from build123d import *

# Parameters (mm, degrees)
ESBO_O1_W                         = 120
ESBO_O1_H                         = 100
ESBO_O1_R                         = 5
RESSALTO_EXTRUS_O1_DEPTH          = 14
REBAIXO_PARA_SHCS_M81_D           = 9
REBAIXO_PARA_SHCS_M81_CBORE_D     = 14
REBAIXO_PARA_SHCS_M81_CBORE_DEPTH = 9


with BuildPart() as part:
    # Esboço1 → Ressalto-extrusão1 (new body)
    with BuildSketch(Plane(origin=(0, 0, 0), x_dir=(1, 0, 0), z_dir=(0, 1, 0))):
        Rectangle(ESBO_O1_W, ESBO_O1_H)
        with Locations(Location((0, 0, 0), (0, 0, 270))):  # turned: the seam where the file's is
            Circle(ESBO_O1_R, mode=Mode.SUBTRACT)
    extrude(amount=RESSALTO_EXTRUS_O1_DEPTH)

    # Rebaixo para SHCS M81 (through all)
    with Locations(Plane(origin=(0, 14, 0), x_dir=(-1, 0, 0), z_dir=(0, 1, 0))):
        with Locations((45, -35), (45, 35), (-45, 35), (-45, -35)):
            CounterBoreHole(REBAIXO_PARA_SHCS_M81_D / 2, REBAIXO_PARA_SHCS_M81_CBORE_D / 2, REBAIXO_PARA_SHCS_M81_CBORE_DEPTH)


solid = part.part
Work out the finished part from the listing and answer in its coordinate system (mm). A direction names the side the tool comes from. Give positions to 0.01 mm unless a question says otherwise; leave off trailing zeros. Order: outer loops, then holes, each group sorted by start corner. A loop starts at its lowest first (then second) coordinate and runs counter-clockwise, first axis right, second up. Notation, with made-up numbers: (5.5, 56.25) -> (24.5, 56.25) arc R19 ccw to (24.5, 64.25) -> close; hole circle Ø9 at (81, 34.25). An arc over 180 degrees is marked (long way). One line per item, written item: value.
Item 1: Find section B-B, the plane x = 45. Give the vertices of the cut face in (y, z).
Answer sheet:
outline: (0, -50) -> (14, -50) -> (14, -42) -> (5, -42) -> (5, -39.5) -> (0, -39.5) -> close; (0, -30.5) -> (5, -30.5) -> (5, -28) -> (14, -28) -> (14, 28) -> (5, 28) -> (5, 30.5) -> (0, 30.5) -> close; (0, 39.5) -> (5, 39.5) -> (5, 42) -> (14, 42) -> (14, 50) -> (0, 50) -> close
Item 2: Flat-ended cylindrical pins translate along their axes: P1, Ø14.5, axis at x = 45, z = 35, coming from the -Y side; P2, Ø4, axis at x = -48.5, z = -35, coming from the +Y side. Find the tip coordinate at first contact, or state that the pin passes through.
Answer sheet:
P1: y = 0
P2: y = 5
Item 3: Find section D-D, the plane y = 3.25. Give the vertices of the cut face in (x, z), plus the area to 3 significant figures.
Answer sheet:
outline: (-60, -50) -> (60, -50) -> (60, 50) -> (-60, 50) -> close; hole circle Ø9 at (-45, -35); hole circle Ø9 at (-45, 35); hole circle Ø10 at (0, 0); hole circle Ø9 at (45, -35); hole circle Ø9 at (45, 35)
area: 11,700 mm²
Item 4: Determine the mould class of faces 1 (the flat face through (-1, 0, 10)), 2 (the flat face through (60, 7, 1)), 3 (the cylindrical face through (-42.92, 2.46, -38.99)) for opening direction X: released by +X, released by -X, zero draft, split by the parting line, or undercut.
Answer sheet:
face 1: zero draft
face 2: released by +X
face 3: undercut
Item 5: Straight lines are drawn through the part: probe 1 along Z at (x, y) = (-45, 2.1); probe 2 along Z at (x, y) = (-45, 7.5); probe 3 along X at (y, z) = (4.5, 0.5). For each, find the intervals that lie inside material, in ascending order.
Answer sheet:
probe 1: -50 to -39.5, -30.5 to 30.5, 39.5 to 50
probe 2: -50 to -42, -28 to 28, 42 to 50
probe 3: -60 to -4.97, 4.97 to 60
Item 6: Find section A-A, the plane z = 0. Give the vertices of the cut face in (x, y).
Answer sheet:
outline: (-60, 0) -> (-5, 0) -> (-5, 14) -> (-60, 14) -> close; (5, 0) -> (60, 0) -> (60, 14) -> (5, 14) -> close
Item 7: Find section C-C, the plane z = -35. Give the vertices of the cut face in (x, y), plus the area to 3 significant figures.
Answer sheet:
outline: (-60, 0) -> (-49.5, 0) -> (-49.5, 5) -> (-52, 5) -> (-52, 14) -> (-60, 14) -> close; (-40.5, 0) -> (40.5, 0) -> (40.5, 5) -> (38, 5) -> (38, 14) -> (-38, 14) -> (-38, 5) -> (-40.5, 5) -> close; (49.5, 0) -> (60, 0) -> (60, 14) -> (52, 14) -> (52, 5) -> (49.5, 5) -> close
area: 1,340 mm²
Item 8: A tool of negligible diameter and unlimited length cuts with its end or side. For faces 4 (the cylindrical face through (47.08, 2.46, -38.99)), 5 (the flat face through (45, 5, 30)), from which of +Z, -Z, +X, -X, +Y, -Y can it reach the whole face along a straight path? Write none if from no direction.
Answer sheet:
face 4: +Y, -Y
face 5: +Y
